```python
from build123d import *

# Parameters (mm, degrees)
SKETCH1_R           = 1.6
BOSS_EXTRUDE1_DEPTH = 5


with BuildPart() as part:
    # Sketch1 → Boss-Extrude1 (new body)
    with BuildSketch(Plane.XY):
        with BuildLine():
            Line((-24.374481213, 29.452498133), (-0.573242194, 29.452498133))
            ThreePointArc((-0.573242194, 29.452498133), (-9.427933785, 33.83519482), (-11.31305575, 43.533643593))
            ThreePointArc((-11.31305575, 43.533643593), (-10.722602644, 61.575298771), (-18.364057527, 77.929445758))
            ThreePointArc((-18.364057527, 77.929445758), (-19.094832363, 82.778042962), (-15.26841437, 85.8442217))
            ThreePointArc((-15.26841437, 85.8442217), (1.199883283, 87.104187108), (17.561282991, 84.846546742))
            ThreePointArc((17.561282991, 84.846546742), (19.39962033, 81.554763647), (18.364057527, 77.929445758))
            ThreePointArc((18.364057527, 77.929445758), (10.722602644, 61.575298771), (11.31305575, 43.533643593))
            ThreePointArc((11.31305575, 43.533643593), (9.427933785, 33.83519482), (0.573242194, 29.452498133))
            Line((0.573242194, 29.452498133), (24.374481213, 29.452498133))
            Line((24.374481213, 29.452498133), (32.479003365, 29.452498133))
            ThreePointArc((32.479003365, 29.452498133), (35.662704371, 31.470373288), (35.196724718, 35.210779041))
            add(Edge.make_bspline(
                [(45.242051564, 75.05397765), (30.132062398, 70.946476879), (22.540088549, 54.680703196), (31.199508073, 39.237934138), (35.196724718, 35.210779041)],
                knots=[0.154808761, 0.154808761, 0.154808761, 0.154808761, 0.468621415, 0.608629265, 0.608629265, 0.608629265, 0.608629265], degree=3))
            ThreePointArc((45.242051564, 75.05397765), (56.35651155, 67.837262053), (66.358030541, 59.143481365))
            ThreePointArc((66.358030541, 59.143481365), (80.500166165, 59.143481365), (80.500166165, 73.285616989))
            ThreePointArc((80.500166165, 73.285616989), (-0.785450823, 106.955221971), (-82.071067812, 73.285616989))
            ThreePointArc((-82.071067812, 73.285616989), (-82.071067758, 59.143481311), (-67.928932081, 59.143481472))
            ThreePointArc((-67.928932081, 59.143481472), (-57.661393829, 68.036973299), (-46.22992721, 75.374419011))
            add(Edge.make_bspline(
                [(-45.055737448, 75), (-46.22992721, 75.374419011)],
                knots=[0, 0, 1, 1], degree=1))
            add(Edge.make_bspline(
                [(-45.055737448, 75), (-29.945748281, 70.892499229), (-22.599492553, 54.774229637), (-31.125849983, 39.411271255), (-35.001982205, 35.428245813)],
                knots=[0.154808761, 0.154808761, 0.154808761, 0.154808761, 0.468621415, 0.60616707, 0.60616707, 0.60616707, 0.60616707], degree=3))
            ThreePointArc((-35.001982205, 35.428245813), (-35.72226494, 31.603661743), (-32.479003365, 29.452498133))
            Line((-32.479003365, 29.452498133), (-24.374481213, 29.452498133))
        make_face()
        with Locations((-22.052924911, 36.483296004)):
            Circle(SKETCH1_R, mode=Mode.SUBTRACT)
        with Locations((-18.364057527, 56.292076909)):
            Circle(SKETCH1_R, mode=Mode.SUBTRACT)
        with Locations((22.052924912, 36.483296004)):
            Circle(SKETCH1_R, mode=Mode.SUBTRACT)
        with Locations((18.364057527, 56.292076909)):
            Circle(SKETCH1_R, mode=Mode.SUBTRACT)
        with Locations((-26.753522246, 73.691170186)):
            Circle(SKETCH1_R, mode=Mode.SUBTRACT)
        with BuildLine():
            ThreePointArc((-80.002588236, 67.275209348), (-1.278913793, 99.883622983), (77.44476065, 67.275209348))
            ThreePointArc((77.44476065, 67.275209348), (77.44476065, 65.153889005), (75.323440307, 65.153889005))
            ThreePointArc((75.323440307, 65.153889005), (-1.278913793, 96.883622983), (-77.881267893, 65.153889005))
            ThreePointArc((-77.881267893, 65.153889005), (-80.002588236, 65.153889005), (-80.002588236, 67.275209348))
        make_face(mode=Mode.SUBTRACT)
        with Locations((26.753522246, 73.691170186)):
            Circle(SKETCH1_R, mode=Mode.SUBTRACT)
    extrude(amount=BOSS_EXTRUDE1_DEPTH)


solid = part.part
```
Here's how the part is built. I have some questions about the finished solid (model axes, mm). A direction names the side the tool comes from. Give positions to 0.01 mm unless a question says otherwise; leave off trailing zeros. Loops run counter-clockwise (first coordinate to the right, second up) from the corner with the lowest first, then second, coordinate; pieces in that order, holes last. Notation, with made-up numbers: M 38,32.5 L 46,32.5 A14 cw 46,45.5 Z; hole C 24.5,22.25 d6. An arc over 180 degrees is marked long. Return JSON: item names as keys, results as strings.
Item 1: Imagine slicing it at C-C on z = 2.6. State how many separate pieces and enclosed holes the cut face has, then the cut area to 3 significant figures.
A:
{"separate pieces": "1", "enclosed holes": "7", "area": "5,210 mm^2"}
Item 2: Imagine slicing it at A-A on y = 89.5. List the corners of the cut face in (x, z) for me, then the cut area to 3 significant figures.
A:
{"outline": "M -61.68,0 L -48.23,0 L -48.23,5 L -61.68,5 Z; M -40.59,0 L 38.03,0 L 38.03,5 L -40.59,5 Z; M 45.67,0 L 60.11,0 L 60.11,5 L 45.67,5 Z", "area": "533 mm^2"}
Item 3: Thinking about a two-plate mould opening in Y: for faces 4 (the cylindrical face through (-57.814, 67.923, 2.465)), 5 (the cylindrical face through (9.514, 33.95, 2.465)), 6 (the cylindrical face through (-9.34, 33.72, 2.46)), 7 (the cylindrical face through (0.48, 106.95, 2.46)), which applies, released by +Y, released by -Y, zero draft, split by the parting line, or undercut?
A:
{"face 4": "released by -Y", "face 5": "undercut", "face 6": "undercut", "face 7": "released by +Y"}
Item 4: Please list where these lines run through material, in increasing order: line 1 (X direction, y = 54.5, z = 4.7); line 2 (X direction, y = 71.5, z = 0.55); line 3 (X direction, y = 66.5, z = 3.3).
A:
{"line 1": "x = -26.77 to -9.94, 9.94 to 26.8", "line 2": "x = -83.49 to -75.54, -70.96 to -52.71, -36.77 to -14.21, 14.21 to 36.86, 51.14 to 68.4, 72.98 to 81.92", "line 3": "x = -85 to -80.41, -76.51 to -59.66, -31.04 to -12.08, 12.08 to 31.14, 58.09 to 73.95, 77.86 to 83.43"}
Item 5: Imagine slicing it at B-B on x = -62.5. List the corners of the cut face in (y, z) for me, then the cut area to 3 significant figures.
A:
{"outline": "M 64.17,0 L 77.93,0 L 77.93,5 L 64.17,5 Z; M 81.54,0 L 88.98,0 L 88.98,5 L 81.54,5 Z", "area": "106 mm^2"}
Item 6: On a 3-axis mill with a long thin cutter (end or side, diameter ignored), from which of +Z, -Z, +X, -X, +Y, -Y can I reach the whole of each face in a straight line? I mean faces 1 (the cylindrical face through (56.208, 67.949, 2.465)), 2 (the flat face through (-21, 77, 0)), 3 (the cylindrical face through (-0.088, 96.877, 2.465)). Say none if no direction works.
A:
{"face 1": "+Z, -Z, -Y", "face 2": "-Z, +X, -X, +Y, -Y", "face 3": "+Z, -Z"}
Item 7: I'm going to push flat-ended pins straight in: pin 1 Ø1 at (y, z) = (78, 4.5) entering from +X (3 decimals); pin 2 Ø3 at (y, z) = (38.5, 4.5) entering from -X. Where does each tip first touch, or does it pass through?
A:
{"pin 1": "stops at x = 76.055", "pin 2": "stops at x = -33.57"}
